from build123d import *

# Parameters (mm, degrees)
ESBO_O1_R                = 10
ESBO_O1_R_2              = 3.25
RESSALTO_EXTRUS_O1_DEPTH = 11
ESBO_O1_3_R              = 3.25
ESBO_O1_3_R_2            = 2.75
RESSALTO_EXTRUS_O2_DEPTH = 12


with BuildPart() as part:
    # Esbo_o1 → Ressalto-extrus_o1 (new, symmetric)
    with BuildSketch(Plane(origin=(0, 0, 0), x_dir=(1, 0, 0), z_dir=(0, 1, 0))):
        with Locations(Location((0, 0, 0), (0, 0, 270))):
            Circle(ESBO_O1_R)
        with Locations(Location((0, 0, 0), (0, 0, 270))):
            Circle(ESBO_O1_R_2, mode=Mode.SUBTRACT)
    extrude(amount=RESSALTO_EXTRUS_O1_DEPTH, both=True)

    # Esbo_o1_3 → Ressalto-extrus_o2 (add, symmetric)
    with BuildSketch(Plane(origin=(0, 0, 0), x_dir=(1, 0, 0), z_dir=(0, 1, 0))):
        with Locations(Location((0, 0, 0), (0, 0, 270))):
            Circle(ESBO_O1_3_R)
        with Locations(Location((0, 0, 0), (0, 0, 270))):
            Circle(ESBO_O1_3_R_2, mode=Mode.SUBTRACT)
    extrude(amount=RESSALTO_EXTRUS_O2_DEPTH, both=True)


solid = part.part
The model under review builds one solid part; all positions refer to its coordinate system, in mm. A direction names the side the tool comes from. Give positions to 0.01 mm unless a question says otherwise; leave off trailing zeros. Order: outer loops, then holes, each group sorted by start corner. A loop starts at its lowest first (then second) coordinate and runs counter-clockwise, first axis right, second up. Notation, with made-up numbers: M 31,-13 L 71,-13 A15 ccw 71,2 Z; hole C -31,82.5 d9. An arc over 180 degrees is marked long. Answer in a Markdown table with one row per item. Add a question column.
1. Add section A-A on z = 0. State the section outline as (x, y) points.
2. For pin 1 Ø2 at (y, z) = (-9, -4.5) entering from +X; pin 2 Ø8 at (x, z) = (7.5, 6.5) entering from +Y; pin 3 Ø10 at (x, y) = (-7.5, -2.5) entering from -Z, all flat-tipped, find the tip position at first contact; note any pin that passes through.
3. To check wall thickness, follow line 1 along X through (y, z) = (0, 0); line 2 along Y through (x, z) = (3.5, -5.25); line 3 along Z through (x, y) = (-0.5, 0). State the ranges of each line that lie inside material, in increasing order.
4. Machinability: for faces 1 (the flat face through (0, -11, 4)), 2 (the cylindrical face through (-9.76, 0.15, -2.17)), 3 (the cylindrical face through (-1.978, 11.507, -2.579)), which of the approach directions +Z, -Z, +X, -X, +Y, -Y give a long, thin tool a straight path to every point of the face, cutting with its end or side? Answer none if there is none.
5. Add section D-D on x = 8. State the section outline as (y, z) points, plus the area to 3 significant figures.
6. Add section B-B on x = 0. State the section outline as (y, z) points, plus the area to 3 significant figures.
7. Mouldability with a two-part tool opening along X and no side actions: class faces 4 (the cylindrical face through (-1.978, -11.493, -2.579)), 5 (the flat face through (0, 11, 4)), 6 (the cylindrical face through (-2.685, -0.168, -0.596)) as released by +X, released by -X, zero draft, split by the parting line, or undercut.
8. Add section C-C on y = 1.5. State the section outline as (x, z) points.
The answers:
| question | item | result |
|---|---|---|
| 1 | outline | M -10,-11 L -3.25,-11 L -3.25,-12 L -2.75,-12 L -2.75,12 L -3.25,12 L -3.25,11 L -10,11 Z; M 2.75,-12 L 3.25,-12 L 3.25,-11 L 10,-11 L 10,11 L 3.25,11 L 3.25,12 L 2.75,12 Z |
| 2 | pin 1 | x = 9.37 |
| 2 | pin 2 | y = 11 |
| 2 | pin 3 | z = -9.68 |
| 3 | line 1 | -10 to -2.75, 2.75 to 10 |
| 3 | line 2 | -11 to 11 |
| 3 | line 3 | -9.99 to -2.7, 2.7 to 9.99 |
| 4 | face 1 | -Y |
| 4 | face 2 | +Y, -Y |
| 4 | face 3 | +Y |
| 5 | outline | M -11,-6 L 11,-6 L 11,6 L -11,6 Z |
| 5 | area | 264 mm2 |
| 6 | outline | M -12,-3.25 L -11,-3.25 L -11,-10 L 11,-10 L 11,-3.25 L 12,-3.25 L 12,-2.75 L -12,-2.75 Z; M -12,2.75 L 12,2.75 L 12,3.25 L 11,3.25 L 11,10 L -11,10 L -11,3.25 L -12,3.25 Z |
| 6 | area | 321 mm2 |
| 7 | face 4 | split by the parting line |
| 7 | face 5 | zero draft |
| 7 | face 6 | undercut |
| 8 | outline | C 0,0 d20; hole C 0,0 d5.5 |
